from build123d import *

# Parameters (mm, degrees)
BOSS_EXTRUDE1_DEPTH = 2
BOSS_EXTRUDE2_DEPTH = 2


with BuildPart() as part:
    # Sketch2 → Boss-Extrude1 (new body)
    with BuildSketch(Plane.XY):
        Polygon((-54.61917065, -24.589230235), (30.72482935, -24.589230235), (13.852659447, -75.725684813), (-71.491340553, -75.725684813), align=None)
    extrude(amount=BOSS_EXTRUDE1_DEPTH)

    # Sketch3 → Boss-Extrude2 (add)
    with BuildSketch(Plane.XY.offset(2)):
        Polygon((-72.764711867, -79.585039875), (11.90144755, -81.639450446), (13.852659447, -75.725684813), (-71.491340553, -75.725684813), align=None)
    extrude(amount=-BOSS_EXTRUDE2_DEPTH)


solid = part.part
Work out the finished part from the listing and answer in its coordinate system (mm). Give positions to 0.01 mm unless a question says otherwise; leave off trailing zeros. Loops run counter-clockwise (first coordinate to the right, second up) from the corner with the lowest first, then second, coordinate; pieces in that order, holes last. Notation, with made-up numbers: (12.25, 1) -> (71.25, 1) arc R25 ccw to (71.25, 34) -> close; hole circle Ø6 at (57.5, 36). An arc over 180 degrees is marked (long way). Use a Markdown table: item, result. Add a question column.
1) The part is cut by section A-A, the plane z = 0.9. Determine the outline of the cut face in (x, y).
2) Consider line 1 along Y through (x, z) = (-8.5, 0.25); line 2 along X through (y, z) = (-73, 1); line 3 along Y through (x, z) = (-28, 0.7). Determine where each line is inside the solid, lowest interval first.
3) The part is cut by section B-B, the plane x = -29. Determine the outline of the cut face in (y, z).
4) The part is cut by section C-C, the plane y = -44. Determine the outline of the cut face in (x, z).
Reported:
| question | item | result |
|---|---|---|
| 1 | outline | (-72.76, -79.59) -> (11.9, -81.64) -> (30.72, -24.59) -> (-54.62, -24.59) -> close |
| 2 | line 1 | y = -81.14 to -24.59 |
| 2 | line 2 | x = -70.59 to 14.75 |
| 2 | line 3 | y = -80.67 to -24.59 |
| 3 | outline | (-80.65, 0) -> (-24.59, 0) -> (-24.59, 2) -> (-80.65, 2) -> close |
| 4 | outline | (-61.02, 0) -> (24.32, 0) -> (24.32, 2) -> (-61.02, 2) -> close |
